Source: three-view drawing plus pictorial views. Frame: mm from the lowest corner of the part. A direction names the side the tool comes from. Round coordinates to 2 decimals unless told otherwise and drop trailing zeros. Order: outer loops, then holes, each group sorted by start corner. A loop starts at its lowest first (then second) coordinate and runs counter-clockwise, first axis right, second up. Notation, with made-up numbers: M -39.5,-14 L -28.5,-14 A15 ccw -28.5,9 Z; hole C 60.5,65 d9. An arc over 180 degrees is marked long. Return JSON: item names as keys, results as strings. Group by question number.
Q1. Cut plane D-D on z = 38.5. Output: boundary loops of the cut face in (x, y).
Q2. Cut plane B-B on z = 6.5. Output: boundary loops of the cut face in (x, y).
Q3. Cut plane C-C on y = 8. Count the separate pieces of the cut face and the enclosed holes in it, and give its area (3 significant figures).
Q4. Ray query, probe 1 along Y at (x, z) = (60.5, 60.5); probe 2 along X at (y, z) = (7.75, 42). Return the intervals inside material, ascending.
Q5. Contact query for a flat-ended pin moving along its axis: pin 1 (8 mm diameter, centred on x = 17, z = 58.5, fed in from +Y). Output: stop coordinate, or through.
Q6. Cut plane A-A on x = 44. Output: boundary loops of the cut face in (y, z).
Q7. Access query for the marked faces 1 and 2. Directions: +Z, -Z, +X, -X, +Y, -Y. A direction counts if a zero-diameter tool reaches every point of the face in a straight line with its end or side. Return the directions, or none.
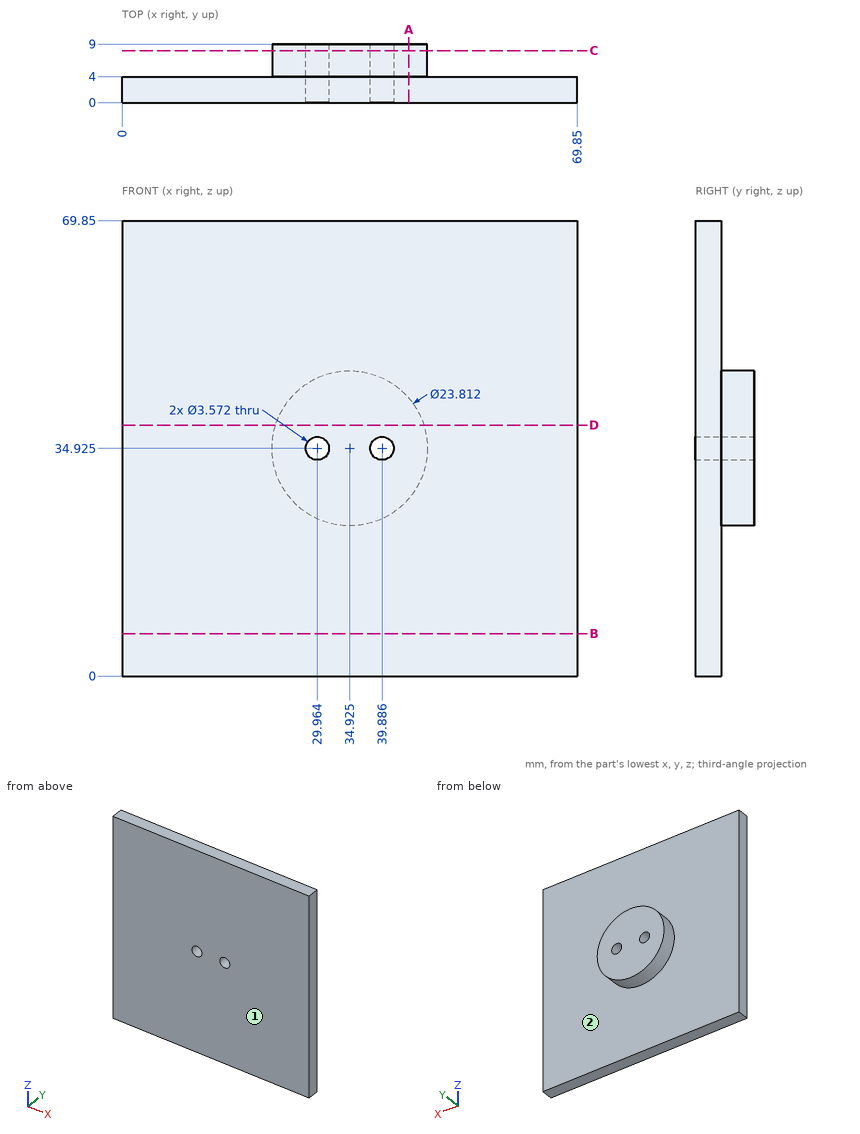
Result sheet:
{
 "1": {"outline": "M 0,0 L 69.85,0 L 69.85,4 L 46.28,4 L 46.28,9 L 23.57,9 L 23.57,4 L 0,4 Z"},
 "2": {"outline": "M 0,0 L 69.85,0 L 69.85,4 L 0,4 Z"},
 "3": {"separate pieces": "1", "enclosed holes": "2", "area": "425 mm²"},
 "4": {"probe 1": "y = 0 to 4", "probe 2": "x = 25.35 to 44.5"},
 "5": {"pin 1": "stops at y = 4"},
 "6": {"outline": "M 0,0 L 4,0 L 4,27.22 L 9,27.22 L 9,42.63 L 4,42.63 L 4,69.85 L 0,69.85 Z"},
 "7": {"face 1": "+Z, -Z, +X, -X, -Y", "face 2": "+Y"}
}
